Check sheet for the modelled part. Datum: model origin and axes. Units: mm. Round coordinates to 2 decimals unless told otherwise and drop trailing zeros. Write each loop counter-clockwise with the first axis right and the second up, starting at its lowest first coordinate (ties: lowest second). Pieces come first, ordered by that corner, then holes. Notation, with made-up numbers: (86, 0.25) -> (121, 0.25) arc R22 cw to (121, 27.25) -> close; hole circle Ø5 at (8, -3). An arc over 180 degrees is marked (long way). One line per item, written item: value.
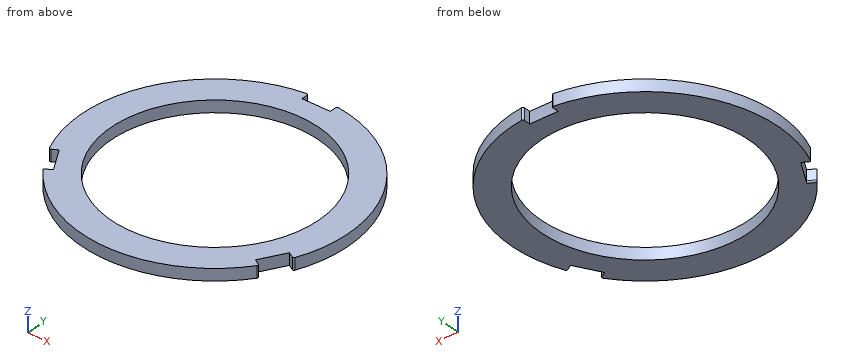
from build123d import *

# Parameters (mm, degrees)
SKETCH1_R           = 17.5
BOSS_EXTRUDE1_DEPTH = 1.984375
FILLET1_R           = 0.25


with BuildPart() as part:
    # Sketch1 → Boss-Extrude1 (new body)
    with BuildSketch(Plane.XY):
        with BuildLine():
            Line((0, 21), (2.38125, 21))
            Line((2.38125, 21), (2.38125, 22.373637354))
            ThreePointArc((2.38125, 22.373637354), (19.485571585, 11.25), (20.566763323, -9.124595684))
            Line((20.566763323, -9.124595684), (19.377158479, -8.437777007))
            Line((19.377158479, -8.437777007), (18.186533479, -10.5))
            Line((18.186533479, -10.5), (16.995908479, -12.562222993))
            Line((16.995908479, -12.562222993), (18.185513323, -13.24904167))
            ThreePointArc((18.185513323, -13.24904167), (0, -22.5), (-18.185513323, -13.24904167))
            Line((-18.185513323, -13.24904167), (-16.995908479, -12.562222993))
            Line((-16.995908479, -12.562222993), (-18.186533479, -10.5))
            Line((-18.186533479, -10.5), (-19.377158479, -8.437777007))
            Line((-19.377158479, -8.437777007), (-20.566763323, -9.124595684))
            ThreePointArc((-20.566763323, -9.124595684), (-19.485571585, 11.25), (-2.38125, 22.373637354))
            Line((-2.38125, 22.373637354), (-2.38125, 21))
            Line((-2.38125, 21), (0, 21))
        make_face()
        Circle(SKETCH1_R, mode=Mode.SUBTRACT)
    extrude(amount=BOSS_EXTRUDE1_DEPTH)

    # Fillet1
    fillet1_edges = [part.edges().sort_by_distance(p)[0] for p in [
        (-17.590710901, -12.905632331, 0),
        (2.38125, 22.373637354, 0.9921875),
        (20.566763323, -9.124595684, 0.9921875),
        (18.185513323, -13.24904167, 0.9921875),
        (-20.566763323, -9.124595684, 0.9921875),
        (-2.38125, 22.373637354, 0.9921875),
    ]]
    fillet(fillet1_edges, radius=FILLET1_R)


solid = part.part
Item 1: Sectioned sample at B-B on x = 0. Enter the section's corners in (y, z).
Answer:
outline: (-22.5, 0) -> (-17.5, 0) -> (-17.5, 1.98) -> (-22.5, 1.98) -> close; (17.5, 0) -> (21, 0) -> (21, 1.98) -> (17.5, 1.98) -> close
Item 2: Sectioned sample at A-A on y = 0. Enter the section's corners in (x, z), and give its area (3 significant figures).
Answer:
outline: (-22.5, 0) -> (-17.5, 0) -> (-17.5, 1.98) -> (-22.5, 1.98) -> close; (17.5, 0) -> (22.5, 0) -> (22.5, 1.98) -> (17.5, 1.98) -> close
area: 19.8 mm^2
Item 3: Sectioned sample at C-C on z = 1.2. Enter the section's corners in (x, y).
Answer:
outline: (-20.68, -8.87) arc R0.25 ccw to (-20.32, -8.98) -> (-19.38, -8.44) -> (-17, -12.56) -> (-18.19, -13.25) arc R22.5 ccw to (18.02, -13.48) arc R0.25 ccw to (17.94, -13.11) -> (17, -12.56) -> (19.38, -8.44) -> (20.32, -8.98) arc R0.25 ccw to (20.68, -8.87) arc R22.5 ccw to (2.66, 22.34) arc R0.25 ccw to (2.38, 22.09) -> (2.38, 21) -> (-2.38, 21) -> (-2.38, 22.09) arc R0.25 ccw to (-2.66, 22.34) arc R22.5 ccw to start; hole circle Ø35 at (0, 0)
Item 4: Thickness scan on line 1 (Y direction, x = 0, z = 0.7); line 2 (X direction, y = -1.5, z = 1.5); line 3 (X direction, y = 14, z = 0.75). Record the ranges inside material, lowest first.
Answer:
line 1: y = -22.5 to -17.5, 17.5 to 21
line 2: x = -22.45 to -17.44, 17.44 to 22.45
line 3: x = -17.61 to -10.5, 10.5 to 17.61
